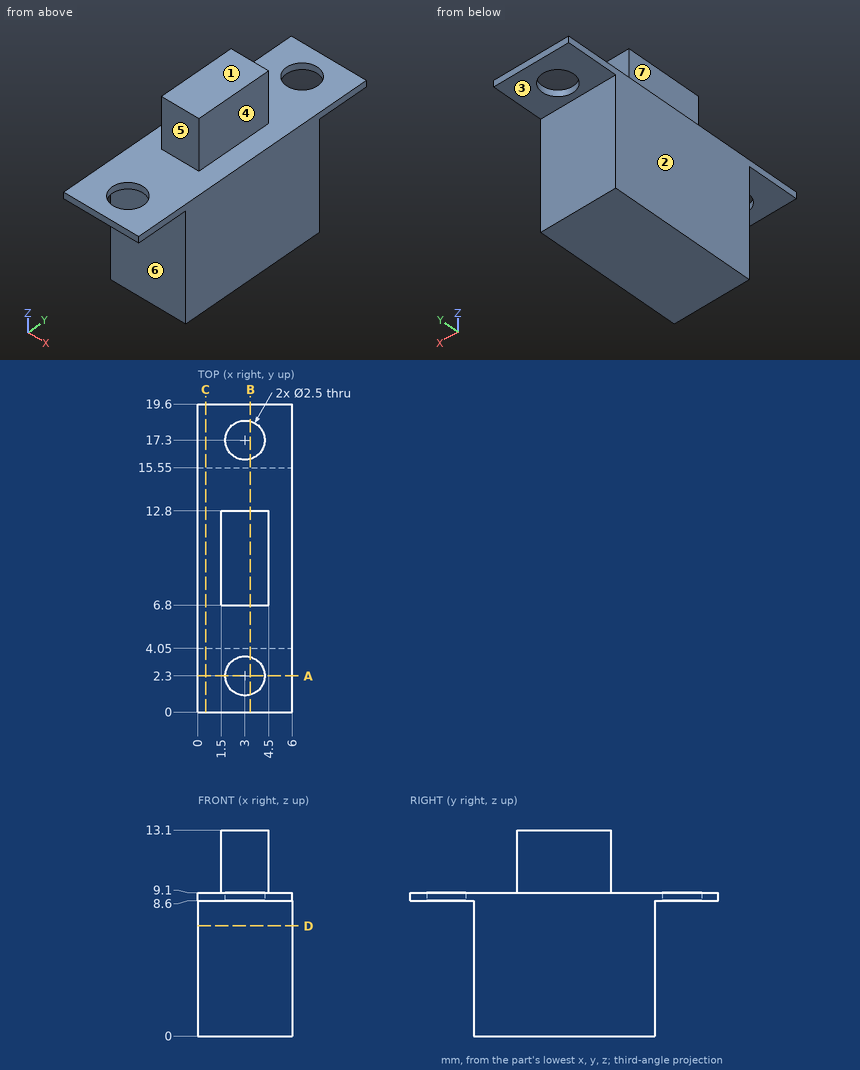
The drawing under review shows one solid part. Ordinate dimensions are in mm from its lowest x, y, z. A direction names the side the tool comes from. Coordinates: 2 decimals unless noted, no trailing zeros. Order: outer loops, then holes, each group sorted by start corner. A loop starts at its lowest first (then second) coordinate and runs counter-clockwise, first axis right, second up. Notation, with made-up numbers: M 56.25,-27.5 L 94.25,-27.5 A29 ccw 94.25,-2.5 Z; hole C 70.5,14.5 d11. An arc over 180 degrees is marked long. Use a Markdown table: item, result.
(1) Add section D-D (z = 7). Give the boundary of the cut face in (x, y).
Worked answers:
| item | result |
|---|---|
| outline | M 0,4.05 L 6,4.05 L 6,15.55 L 0,15.55 Z |
(2) Add section A-A (y = 2.3). Give the boundary of the cut face in (x, z).
Worked answers:
| item | result |
|---|---|
| outline | M 0,8.6 L 1.75,8.6 L 1.75,9.1 L 0,9.1 Z; M 4.25,8.6 L 6,8.6 L 6,9.1 L 4.25,9.1 Z |
(3) Wall thickness on probe 1 along Y at (x, z) = (3, 8.9); probe 2 along Y at (x, z) = (1.5, 7); probe 3 along Z at (x, y) = (5.5, 5.5): over which ranges is each line inside the solid? List them lowest first.
Worked answers:
| item | result |
|---|---|
| probe 1 | y = 0 to 1.05, 3.55 to 16.05, 18.55 to 19.6 |
| probe 2 | y = 4.05 to 15.55 |
| probe 3 | z = 0 to 9.1 |
(4) Add section B-B (x = 3.35). Give the boundary of the cut face in (y, z).
Worked answers:
| item | result |
|---|---|
| outline | M 0,8.6 L 1.1,8.6 L 1.1,9.1 L 0,9.1 Z; M 3.5,8.6 L 4.05,8.6 L 4.05,0 L 15.55,0 L 15.55,8.6 L 16.1,8.6 L 16.1,9.1 L 12.8,9.1 L 12.8,13.1 L 6.8,13.1 L 6.8,9.1 L 3.5,9.1 Z; M 18.5,8.6 L 19.6,8.6 L 19.6,9.1 L 18.5,9.1 Z |
(5) For P1, Ø3, axis at x = 1, y = 3, coming from the +Z side; P2, Ø0.9, axis at x = 3, z = 10, coming from the -Y side; P3, Ø3, axis at y = 10.5, z = 12, coming from the +X side; P4, Ø2, axis at x = 3, y = 2.3, coming from the +Z side, all flat-tipped, find the tip position at first contact; note any pin that passes through.
Worked answers:
| item | result |
|---|---|
| P1 | stops at z = 9.1 |
| P2 | stops at y = 6.8 |
| P3 | stops at x = 4.5 |
| P4 | passes through |
(6) Add section C-C (x = 0.5). Give the boundary of the cut face in (y, z), then the cut area to 3 significant figures.
Worked answers:
| item | result |
|---|---|
| outline | M 0,8.6 L 4.05,8.6 L 4.05,0 L 15.55,0 L 15.55,8.6 L 19.6,8.6 L 19.6,9.1 L 0,9.1 Z |
| area | 109 mm2 |
(7) Draft analysis for pull direction Z (two halves, no side actions). For the marked faces 1, 2 and 3, state which applies: released by +Z, released by -Z, zero draft, split by the parting line, or undercut.
Worked answers:
| item | result |
|---|---|
| face 1 | released by +Z |
| face 2 | zero draft |
| face 3 | released by -Z |
(8) For the marked faces 4, 5, 6 and 7, list the 3-axis set-ups (+Z, -Z, +X, -X, +Y, -Y) from which the entire face can be reached by the end or side of a thin tool; tool diameter is ignored.
Worked answers:
| item | result |
|---|---|
| face 4 | +Z, +X, +Y, -Y |
| face 5 | +Z, +X, -X, -Y |
| face 6 | -Z, +X, -X, -Y |
| face 7 | +Z, -X, +Y, -Y |
